```python
from build123d import *

# Parameters (mm, degrees)
BOSS_EXTRUDE1_DEPTH = 45
CUT_EXTRUDE1_DEPTH  = 45


with BuildPart() as part:
    # Sketch1 → Boss-Extrude1 (new body)
    with BuildSketch(Plane(origin=(0, 0, 0), x_dir=(0, 0, -1), z_dir=(1, 0, 0))):
        Polygon((0, 0), (27, 0), (27, 10), (19.5, 10), (19.5, 4), (7.5, 4), (7.5, 10), (0, 10), align=None)
    extrude(amount=BOSS_EXTRUDE1_DEPTH)

    # Sketch2 → Cut-Extrude1 (cut)
    with BuildSketch(Plane.XZ):
        with BuildLine():
            ThreePointArc((31, -3.5), (31.439339828, -4.560660172), (32.5, -5))
            Line((32.5, -5), (32.5, -3.5))
            Line((32.5, -3.5), (31, -3.5))
        make_face()
        with BuildLine():
            Line((32.5, -3.5), (32.5, -5))
            ThreePointArc((32.5, -5), (33.560660172, -4.560660172), (34, -3.5))
            ThreePointArc((34, -3.5), (32.5, -2), (31, -3.5))
            Line((31, -3.5), (32.5, -3.5))
        make_face()
        with BuildLine():
            ThreePointArc((32.5, -22), (31.439339828, -22.439339828), (31, -23.5))
            Line((31, -23.5), (32.5, -23.5))
            Line((32.5, -23.5), (32.5, -22))
        make_face()
        with BuildLine():
            Line((32.5, -23.5), (31, -23.5))
            ThreePointArc((31, -23.5), (32.5, -25), (34, -23.5))
            ThreePointArc((34, -23.5), (33.560660172, -22.439339828), (32.5, -22))
            Line((32.5, -22), (32.5, -23.5))
        make_face()
        with BuildLine():
            Line((12.5, -22), (12.5, -23.5))
            Line((12.5, -23.5), (14, -23.5))
            ThreePointArc((14, -23.5), (13.560660172, -22.439339828), (12.5, -22))
        make_face()
        with BuildLine():
            Line((14, -23.5), (12.5, -23.5))
            Line((12.5, -23.5), (12.5, -22))
            ThreePointArc((12.5, -22), (11.439339828, -24.560660172), (14, -23.5))
        make_face()
        with BuildLine():
            ThreePointArc((14, -3.5), (11.439339828, -2.439339828), (12.5, -5))
            Line((12.5, -5), (12.5, -3.5))
            Line((12.5, -3.5), (14, -3.5))
        make_face()
        with BuildLine():
            Line((12.5, -3.5), (12.5, -5))
            ThreePointArc((12.5, -5), (13.560660172, -4.560660172), (14, -3.5))
            Line((14, -3.5), (12.5, -3.5))
        make_face()
    extrude(amount=-CUT_EXTRUDE1_DEPTH, mode=Mode.SUBTRACT)


solid = part.part
```
For this review, take the finished solid that the model builds, in its own axes (mm). A direction names the side the tool comes from. Give positions to 0.01 mm unless a question says otherwise; leave off trailing zeros. Write each loop counter-clockwise with the first axis right and the second up, starting at its lowest first coordinate (ties: lowest second). Pieces come first, ordered by that corner, then holes. Notation, with made-up numbers: M 81,-3.5 L 97,-3.5 A27 ccw 97,21.5 Z; hole C 42.5,-25 d6. An arc over 180 degrees is marked long. One line per item, written item: value.
1) Take a section at D-D, the plane y = 3.5. Write out the cut boundary in (x, z), then the cut area to 3 significant figures.
Results are:
outline: M 0,-27 L 45,-27 L 45,0 L 0,0 Z; hole C 12.5,-23.5 d3; hole C 12.5,-3.5 d3; hole C 32.5,-23.5 d3; hole C 32.5,-3.5 d3
area: 1,190 mm²
2) Take a section at B-B, the plane z = -24.5. Write out the cut boundary in (x, y).
Results are:
outline: M 0,0 L 11.38,0 L 11.38,10 L 0,10 Z; M 13.62,0 L 31.38,0 L 31.38,10 L 13.62,10 Z; M 33.62,0 L 45,0 L 45,10 L 33.62,10 Z
3) Take a section at C-C, the plane x = 40.5. Write out the cut boundary in (y, z).
Results are:
outline: M 0,-27 L 10,-27 L 10,-19.5 L 4,-19.5 L 4,-7.5 L 10,-7.5 L 10,0 L 0,0 Z
4) The part is to be moulded in two halves that separate along Z. For faces 3 (the flat face through (22, 4, -14)), 4 (the flat face through (22, 5, 0)), 5 (the flat face through (0, 3, -13)), 6 (the flat face through (22, 7, -7.5)), say which applies: +Z half, -Z half, draft (parallel to the pull), parting line (faces both ways), or undercut.
Results are:
face 3: undercut
face 4: +Z half
face 5: draft
face 6: undercut
5) Take a section at A-A, the plane y = 7. Write out the cut boundary in (x, z).
Results are:
outline: M 0,-27 L 45,-27 L 45,-19.5 L 0,-19.5 Z; M 0,-7.5 L 45,-7.5 L 45,0 L 0,0 Z; hole C 12.5,-23.5 d3; hole C 12.5,-3.5 d3; hole C 32.5,-23.5 d3; hole C 32.5,-3.5 d3
6) For line 1 (Z direction, x = 12.5, y = 6.5); line 2 (X direction, y = 6.25, z = -23.5); line 3 (Z direction, x = 12.5, y = 2.75), list the stretches that pass through material, from the lowest coordinate up. Write a range as from..to.
Results are:
line 1: z = -27..-25, -22..-19.5, -7.5..-5, -2..0
line 2: x = 0..11, 14..31, 34..45
line 3: z = -27..-25, -22..-5, -2..0
7) For P1, Ø3.5, axis at x = 16, z = -16, coming from the +Y side, flat-tipped, find the tip position at first contact; note if it passes through.
Results are:
P1: stops at y = 4
8) For faces 1 (the flat face through (45, 3, -13)), 2 (the flat face through (22, 7, -19.5)), list the 3-axis set-ups (+Z, -Z, +X, -X, +Y, -Y) from which the entire face can be reached by the end or side of a thin tool; tool diameter is ignored.
Results are:
face 1: +Z, -Z, +X, +Y, -Y
face 2: +X, -X, +Y
